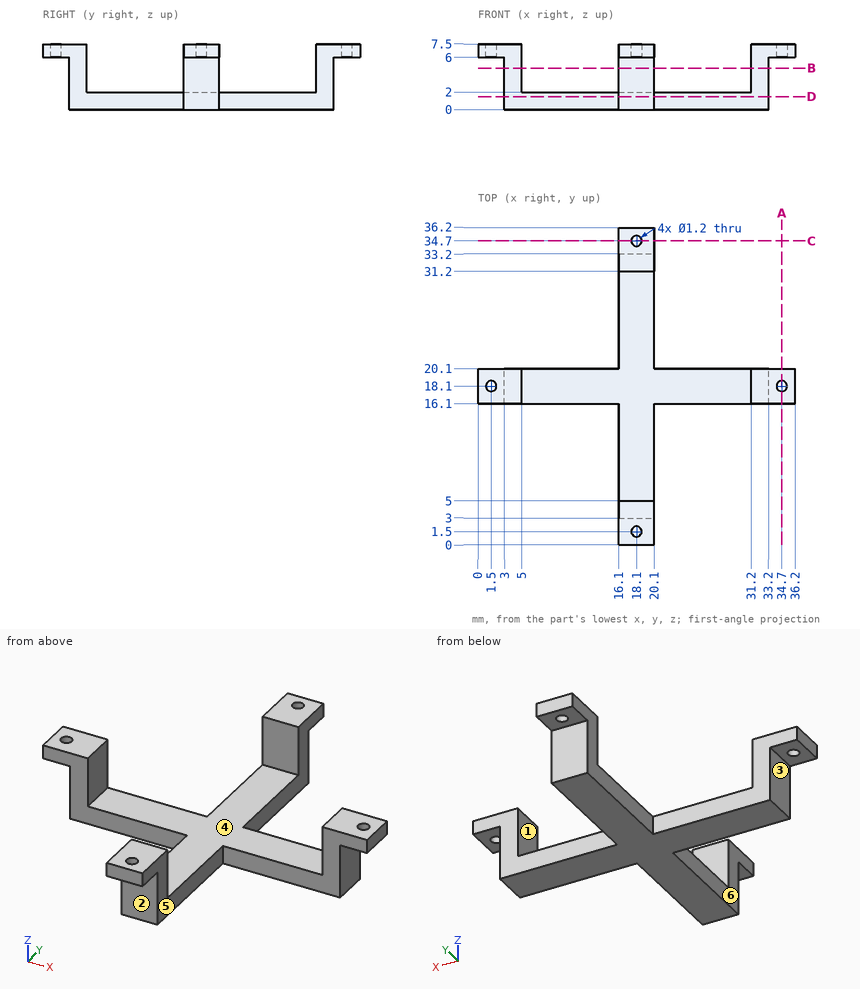
Drawing for the job (mm, zero at the part's lowest x, y, z). A direction names the side the tool comes from. Give positions to 0.01 mm unless a question says otherwise; leave off trailing zeros. Order: outer loops, then holes, each group sorted by start corner. A loop starts at its lowest first (then second) coordinate and runs counter-clockwise, first axis right, second up. Notation, with made-up numbers: (-23, 22) - (33, 22) arc R11 ccw to (33, 43) - close; hole circle Ø8 at (40, 16). An arc over 180 degrees is marked (long way). Write item = value, one per line. Start each with the question number.
1. Cut at A-A, the plane x = 34.7. List the corners of the cut face in (y, z).
2. Cut at D-D, the plane z = 1.5. List the corners of the cut face in (x, y), and give its area (3 significant figures).
3. Two-plate mould, pull along X, no slides. Class the marked faces 1, 2 and 3: pulls with the +X half, pulls with the -X half, needs draft (parallel to the pull), parting line crosses it, or undercut.
4. Cut at B-B, the plane z = 4.75. List the corners of the cut face in (x, y), and give its area (3 significant figures).
5. Probe line 1 along Y through (x, z) = (18.1, 6.65); line 2 along Y through (x, z) = (1.5, 6.45). List the from-to ranges inside material, lowest first.
6. Which spindle directions (+Z, -Z, +X, -X, +Y, -Y) get a long thin tool onto all of the face, cutting with end or side? Do the marked faces 4, 5 and 6. Say none if no direction does.
7. Drop flat-ended pins along their axis: P1, Ø1.4, axis at x = 18.1, y = 1.5, coming from the -Z side; P2, Ø4, axis at y = 10, z = 3, coming from the -X side; P3, Ø4.5, axis at y = 17.5, z = 2.5, coming from the -X side; P4, Ø2, axis at x = 29, z = 4, coming from the +Y side. Give the stop position or say it passes through.
Taken from the geometry:
q1.outline = (16.1, 6) - (17.5, 6) - (17.5, 7.5) - (16.1, 7.5) - close; (18.7, 6) - (20.1, 6) - (20.1, 7.5) - (18.7, 7.5) - close
q2.outline = (3, 16.1) - (16.1, 16.1) - (16.1, 3) - (20.1, 3) - (20.1, 16.1) - (33.2, 16.1) - (33.2, 20.1) - (20.1, 20.1) - (20.1, 33.2) - (16.1, 33.2) - (16.1, 20.1) - (3, 20.1) - close
q2.area = 226 mm²
q3.face_1 = undercut
q3.face_2 = needs draft
q3.face_3 = pulls with the -X half
q4.outline = (3, 16.1) - (5, 16.1) - (5, 20.1) - (3, 20.1) - close; (16.1, 3) - (20.1, 3) - (20.1, 5) - (16.1, 5) - close; (16.1, 31.2) - (20.1, 31.2) - (20.1, 33.2) - (16.1, 33.2) - close; (31.2, 16.1) - (33.2, 16.1) - (33.2, 20.1) - (31.2, 20.1) - close
q4.area = 32.0 mm²
q5.line_1 = 0 to 0.9, 2.1 to 5, 31.2 to 34.1, 35.3 to 36.2
q5.line_2 = 16.1 to 17.5, 18.7 to 20.1
q6.face_4 = +Z
q6.face_5 = +Z, -Z, +X, -Y
q6.face_6 = +Z, -Z, -X, -Y
q7.P1 = 6
q7.P2 = 16.1
q7.P3 = 3
q7.P4 = through
